CAD build for the part. Positions are in the model's coordinates, mm. A direction names the side the tool comes from. Round coordinates to 2 decimals unless told otherwise and drop trailing zeros. Order: outer loops, then holes, each group sorted by start corner. A loop starts at its lowest first (then second) coordinate and runs counter-clockwise, first axis right, second up. Notation, with made-up numbers: M 78,66 L 87,66 A23 ccw 87,89 Z; hole C -6,49 d9. An arc over 180 degrees is marked long. Answer as a JSON object with one key per item and string values.
```python
from build123d import *

# Parameters (mm, degrees)
F0_W     = 20
F0_H     = 20
F1_DEPTH = 5
F2_DEPTH = 2
F4_D     = 5.5


with BuildPart() as f1:
    # F0 (on Top) → F1 (new body)
    with BuildSketch(Plane.XY):
        Polygon((10, 10), (-30, 10), (-30, -10), (-7.5, -10), (-7.5, -7), (7.5, -7), (7.5, -10), (10, -10), align=None)
        with Locations((20, 0)):
            Rectangle(F0_W, F0_H)
    extrude(amount=-F1_DEPTH)

    # F0 (on Top) → F2 (join)
    with BuildSketch(Plane.XY):
        with Locations((20, 0)):
            Rectangle(F0_W, F0_H)
    extrude(amount=F2_DEPTH)

    # F4 (through all)
    with Locations(Plane(origin=(0, 0, -5), x_dir=(1, 0, 0), z_dir=(0, 0, -1))):
        with Locations((-20, 0), (20, 0), (-4, 0)):
            Hole(F4_D / 2)


solid = f1.part
```
Item 1: Drop flat-ended pins along their axis: pin 1 Ø4 at (x, z) = (1.5, -3) entering from -Y; pin 2 Ø3.5 at (x, y) = (20, 0) entering from +Z; pin 3 Ø8 at (x, y) = (-18, 7) entering from +Z; pin 4 Ø6.5 at (x, y) = (-4, 0) entering from -Z. Give the stop position or say it passes through.
Worked answers:
{"pin 1": "stops at y = -7", "pin 2": "passes through", "pin 3": "stops at z = 0", "pin 4": "stops at z = -5"}
Item 2: Saw through at A-A on x = -20. List the corners of the cut face in (y, z), and give its area (3 significant figures).
Worked answers:
{"outline": "M -10,-5 L -2.75,-5 L -2.75,0 L -10,0 Z; M 2.75,-5 L 10,-5 L 10,0 L 2.75,0 Z", "area": "72.5 mm2"}
Item 3: Saw through at B-B on z = -2. List the corners of the cut face in (x, y), and give its area (3 significant figures).
Worked answers:
{"outline": "M -30,-10 L -7.5,-10 L -7.5,-7 L 7.5,-7 L 7.5,-10 L 30,-10 L 30,10 L -30,10 Z; hole C -20,0 d5.5; hole C -4,0 d5.5; hole C 20,0 d5.5", "area": "1,080 mm2"}
Item 4: Wall check: line 1 along X through (y, z) = (-7.5, -4); line 2 along Y through (x, z) = (20, -2.5); line 3 along X through (y, z) = (3.5, 0.25). Give the ranges that are in metal, low to high. Write a range as [from, to].
Worked answers:
{"line 1": "x = [-30, -7.5], [7.5, 30]", "line 2": "y = [-10, -2.75], [2.75, 10]", "line 3": "x = [10, 30]"}
Item 5: Saw through at D-D on z = 1.25. List the corners of the cut face in (x, y).
Worked answers:
{"outline": "M 10,-10 L 30,-10 L 30,10 L 10,10 Z; hole C 20,0 d5.5"}
Item 6: 3-axis set-ups, long thin cutter, end or side, ignore diameter. For faces 1 (the flat face through (-30, 0, -2)), 2 (the flat face through (-7.5, -9, -2)), 3 (the flat face through (10, 0, 1)): which of +Z, -Z, +X, -X, +Y, -Y reach the whole face in a straight line?
Worked answers:
{"face 1": "+Z, -Z, -X, +Y, -Y", "face 2": "+Z, -Z, -Y", "face 3": "+Z, -X, +Y, -Y"}
Item 7: Two-plate mould, pull along Y, no slides. Class faces 4 (the flat face through (7.5, -8, -2)), 5 (the flat face through (-19, -10, -2)), 6 (the flat face through (0, 10, -2)), 7 (the cylindrical face through (22.747, -0.121, -1.451)): released by +Y, released by -Y, zero draft, split by the parting line, or undercut.
Worked answers:
{"face 4": "zero draft", "face 5": "released by -Y", "face 6": "released by +Y", "face 7": "undercut"}
Item 8: Saw through at C-C on y = 0. List the corners of the cut face in (x, z), and give its area (4 significant figures).
Worked answers:
{"outline": "M -30,-5 L -22.75,-5 L -22.75,0 L -30,0 Z; M -17.25,-5 L -6.75,-5 L -6.75,0 L -17.25,0 Z; M -1.25,-5 L 17.25,-5 L 17.25,2 L 10,2 L 10,0 L -1.25,0 Z; M 22.75,-5 L 30,-5 L 30,2 L 22.75,2 Z", "area": "246.5 mm2"}
